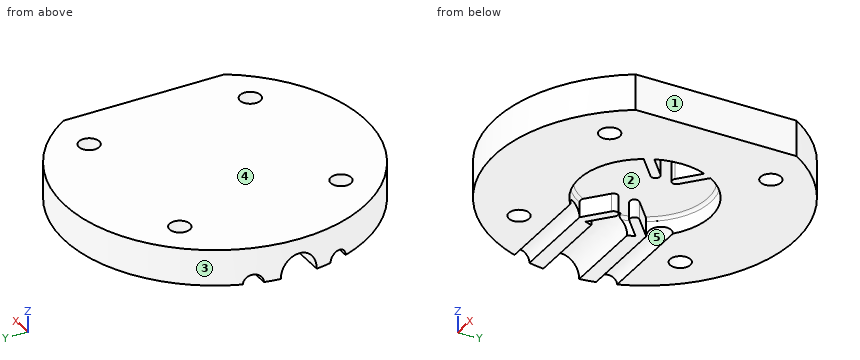
from build123d import *

# Parameters (mm, degrees)
ESQUISSE1_R             = 25
ESQUISSE1_R_2           = 1.7
BOSS_EXTRU_1_DEPTH      = 6
ESQUISSE6_R             = 11
ENL_V_MAT_EXTRU_2_DEPTH = 3
CONG_2_R                = 0.5
BOSS_EXTRU_6_DEPTH      = 6
ESQUISSE12_RX           = 3.57944127
ESQUISSE12_RY           = 3
ENL_V_MAT_EXTRU_3_DEPTH = 15
ESQUISSE13_W            = 18.660647855
ESQUISSE13_H            = 1.5
ESQUISSE14_W            = 18.40878356
ESQUISSE14_H            = 1.5
ESQUISSE15_W            = 7.963879273
ESQUISSE15_H            = 27.450042448
ENL_V_MAT_EXTRU_4_DEPTH = 36.860842729


with BuildPart() as part:
    # Esquisse1 → Boss.-Extru.1 (new body)
    with BuildSketch(Plane.XY):
        Circle(ESQUISSE1_R)
        with Locations((-13.435028843, 13.435028843)):
            Circle(ESQUISSE1_R_2, mode=Mode.SUBTRACT)
        with Locations((13.435028843, 13.435028843)):
            Circle(ESQUISSE1_R_2, mode=Mode.SUBTRACT)
        with Locations((13.435028843, -13.435028843)):
            Circle(ESQUISSE1_R_2, mode=Mode.SUBTRACT)
        with Locations((-13.435028843, -13.435028843)):
            Circle(ESQUISSE1_R_2, mode=Mode.SUBTRACT)
    extrude(amount=BOSS_EXTRU_1_DEPTH)

    # Esquisse6 → Enlèv. mat.-Extru.2 (cut)
    with BuildSketch(Plane(origin=(0, 0, 0), x_dir=(-1, 0, 0), z_dir=(0, 0, -1))):
        Circle(ESQUISSE6_R)
    extrude(amount=-ENL_V_MAT_EXTRU_2_DEPTH, mode=Mode.SUBTRACT)

    # Congé2
    cong_2_edges = [part.edges().sort_by_distance(p)[0] for p in [
        (11, 0, 3),
    ]]
    fillet(cong_2_edges, radius=CONG_2_R)

    # Esquisse10 → Boss.-Extru.6 (add)
    with BuildSketch(Plane.XY.offset(6)):
        with BuildLine():
            Line((-5.758802096, -2.316766812), (-9.508802096, -5.566766812))
            ThreePointArc((-9.508802096, -5.566766812), (-10.566766812, -5.491197904), (-10.491197904, -4.433233188))
            Line((-10.491197904, -4.433233188), (-6.741197904, -1.183233188))
            ThreePointArc((-6.741197904, -1.183233188), (-5.683233188, -1.258802096), (-5.758802096, -2.316766812))
        make_face()
        with BuildLine():
            Line((-6.741197904, 1.183233188), (-10.491197904, 4.433233188))
            ThreePointArc((-10.491197904, 4.433233188), (-10.566766812, 5.491197904), (-9.508802096, 5.566766812))
            Line((-9.508802096, 5.566766812), (-5.758802096, 2.316766812))
            ThreePointArc((-5.758802096, 2.316766812), (-5.683233188, 1.258802096), (-6.741197904, 1.183233188))
        make_face()
        with BuildLine():
            Line((9.508802096, -5.566766812), (5.758802096, -2.316766812))
            ThreePointArc((5.758802096, -2.316766812), (5.683233188, -1.258802096), (6.741197904, -1.183233188))
            Line((6.741197904, -1.183233188), (10.491197904, -4.433233188))
            ThreePointArc((10.491197904, -4.433233188), (10.566766812, -5.491197904), (9.508802096, -5.566766812))
        make_face()
        with BuildLine():
            Line((10.491197904, 4.433233188), (6.741197904, 1.183233188))
            ThreePointArc((6.741197904, 1.183233188), (5.683233188, 1.258802096), (5.758802096, 2.316766812))
            Line((5.758802096, 2.316766812), (9.508802096, 5.566766812))
            ThreePointArc((9.508802096, 5.566766812), (10.566766812, 5.491197904), (10.491197904, 4.433233188))
        make_face()
    extrude(amount=-BOSS_EXTRU_6_DEPTH)

    # Esquisse12 → Enlèv. mat.-Extru.3 (cut)
    with BuildSketch(Plane.ZY.offset(25)):
        with Locations(Location((0, 0), (0, 0, 180))):
            Ellipse(ESQUISSE12_RX, ESQUISSE12_RY)
    extrude(amount=-ENL_V_MAT_EXTRU_3_DEPTH, mode=Mode.SUBTRACT)

    # Esquisse13 → Enlèvement de matière-Révolution1 (revolve, cut)
    with BuildSketch(Plane(origin=(0, 0, 0), x_dir=(-1, 0, 0), z_dir=(0, 0, -1))):
        with Locations((15.635249349, 6.304475395)):
            Rectangle(ESQUISSE13_W, ESQUISSE13_H)
    revolve(axis=Axis((-24.965573276, 7.054475395, 0), (1, 0, 0)), mode=Mode.SUBTRACT)

    # Esquisse14 → Enlèvement de matière-Révolution2 (revolve, cut)
    with BuildSketch(Plane(origin=(0, 0, 0), x_dir=(-1, 0, 0), z_dir=(0, 0, -1))):
        with Locations((15.170755462, -6.304475395)):
            Rectangle(ESQUISSE14_W, ESQUISSE14_H)
    revolve(axis=Axis((-24.375147242, -7.054475395, 0), (1, 0, 0)), mode=Mode.SUBTRACT)

    # Esquisse15 → Enlèv. mat.-Extru.4 (cut, through all)
    with BuildSketch(Plane(origin=(0, 0, 0), x_dir=(-1, 0, 0), z_dir=(0, 0, -1))):
        with Locations((-25.065108278, -0.289992381)):
            Rectangle(ESQUISSE15_W, ESQUISSE15_H)
    extrude(amount=-ENL_V_MAT_EXTRU_4_DEPTH, mode=Mode.SUBTRACT)


solid = part.part
Could you check a few things on this model? Use its own coordinates, in mm. Face numbers are marked on the shaded views. A direction names the side the tool comes from. Give positions to 0.01 mm unless a question says otherwise; leave off trailing zeros. Order: outer loops, then holes, each group sorted by start corner. A loop starts at its lowest first (then second) coordinate and runs counter-clockwise, first axis right, second up.
1. Suppose I cut it at D-D (y = -19.5). List the corners of the cut face in (x, z) for me, plus the area to 3 significant figures.
2. Will these pins go through, and if not, where does the flat tip stop? P1, Ø1.5, axis at y = 7.5, z = 1, coming from the -X side; P2, Ø3, axis at x = 13.44, y = 13.44, coming from the +Z side.
3. Suppose I cut it at A-A (x = 0). List the corners of the cut face in (y, z) for me, plus the area to 3 significant figures.
4. Suppose I cut it at C-C (z = 4.5). List the corners of the cut face in (x, y) for me, plus the area to 3 significant figures.
5. We'd pull the mould along Y, two halves only. Please class the marked faces 3, 4 and 5: pulls with the +Y half, pulls with the -Y half, needs draft (parallel to the pull), parting line crosses it, or undercut.
6. For the marked faces 1 and 2, which set-ups out of +Z, -Z, +X, -X, +Y, -Y let a thin tool reach every point of the face, with its end or its side?
7. I need wall thicknesses on L1, parallel to X at y = 12, z = 1; L2, parallel to Y at x = 6, z = 0.75; L3, parallel to Z at x = 1, y = 6. Which ranges of each line are inside material? Lowest first, please.
8. Suppose I cut it at B-B (y = 14). List the corners of the cut face in (x, z) for me, plus the area to 3 significant figures.
Solved:
1. outline: (-15.64, 0) - (15.64, 0) - (15.64, 6) - (-15.64, 6) - close
1. area: 188 mm2
2. P1: stops at x = -24.02
2. P2: passes through
3. outline: (-25, 0) - (-11, 0) - (-11, 2.5) arc R0.5 cw to (-10.5, 3) - (10.5, 3) arc R0.5 cw to (11, 2.5) - (11, 0) - (25, 0) - (25, 6) - (-25, 6) - close
3. area: 234 mm2
4. outline: (21.08, -13.44) - (21.08, 13.44) arc R25 ccw (long way) to start; hole circle Ø3.4 at (-13.44, -13.44); hole circle Ø3.4 at (-13.44, 13.44); hole circle Ø3.4 at (13.44, -13.44); hole circle Ø3.4 at (13.44, 13.44)
4. area: 1,860 mm2
5. face 3: parting line crosses it
5. face 4: needs draft
5. face 5: undercut
6. face 1: +Z, -Z, +X, +Y, -Y
6. face 2: -Z
7. L1: x = -21.93 to -14.35, -12.52 to 12.52, 14.35 to 21.08
7. L2: y = -24.27 to -9.22, -2.53 to -1.04, 1.04 to 2.53, 9.22 to 24.27
7. L3: z = 3 to 6
8. outline: (-20.71, 0) - (-15.04, 0) - (-15.04, 6) - (-20.71, 6) - close; (-11.83, 0) - (11.83, 0) - (11.83, 6) - (-11.83, 6) - close; (15.04, 0) - (20.71, 0) - (20.71, 6) - (15.04, 6) - close
8. area: 210 mm2
